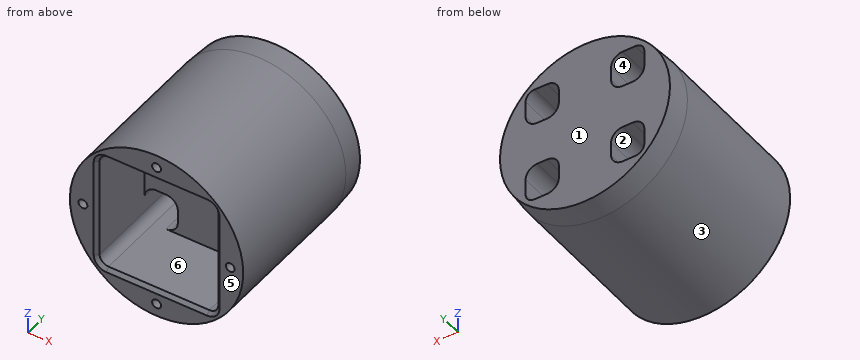
from build123d import *

# Parameters (mm, degrees)
SKETCH2_R           = 73.75
MAINDOUGHNUT_DEPTH  = 150
SKETCH3_R           = 3.81
CUT_EXTRUDE1_DEPTH  = 183.696811685
NOSECONETAPER_SIZE  = 20
NOSECONETAPER_SIZE2 = 1.398536239
PAYLOADSTOPS_DEPTH  = 90
FILLET1_R           = 10
FILLET2_R           = 10
FILLET3_R           = 10
CHAMFER1_SIZE       = 3


with BuildPart() as part:
    # Sketch2 → MainDoughnut (new body)
    with BuildSketch(Plane(origin=(0, 0, 0), x_dir=(1, 0, 0), z_dir=(0, 1, 0))):
        with Locations(Location((0, 0, 0), (0, 0, 270))):
            Circle(SKETCH2_R)
        with BuildLine():
            Line((42.87, -50.5), (-42.87, -50.5))
            ThreePointArc((-42.87, -50.5), (-48.26522474, -48.26522474), (-50.5, -42.87))
            Line((-50.5, -42.87), (-50.5, 42.87))
            ThreePointArc((-50.5, 42.87), (-48.26522474, 48.26522474), (-42.87, 50.5))
            Line((-42.87, 50.5), (42.87, 50.5))
            ThreePointArc((42.87, 50.5), (48.26522474, 48.26522474), (50.5, 42.87))
            Line((50.5, 42.87), (50.5, -42.87))
            ThreePointArc((50.5, -42.87), (48.26522474, -48.26522474), (42.87, -50.5))
        make_face(mode=Mode.SUBTRACT)
    extrude(amount=MAINDOUGHNUT_DEPTH)

    # Sketch3 → Cut-Extrude1 (cut, through all)
    with BuildSketch(Plane(origin=(0, 150, 0), x_dir=(1, 0, 0), z_dir=(0, 1, 0))):
        with Locations(Location((-62.711477498, 0, 0), (0, 0, 270))):
            Circle(SKETCH3_R)
        with Locations(Location((0, 62.711477498, 0), (0, 0, 270))):
            Circle(SKETCH3_R)
        with Locations(Location((62.711477498, 0, 0), (0, 0, 270))):
            Circle(SKETCH3_R)
        with Locations(Location((0, -62.711477498, 0), (0, 0, 270))):
            Circle(SKETCH3_R)
    extrude(amount=-CUT_EXTRUDE1_DEPTH, mode=Mode.SUBTRACT)

    # NoseconeTaper
    noseconetaper_edges = [part.edges().sort_by_distance(p)[0] for p in [
        (0, 150, -73.75),
    ]]
    noseconetaper_side = [part.faces().sort_by_distance(p)[0] for p in [
        (0, 75, -73.75),
    ]]
    chamfer(noseconetaper_edges, length=NOSECONETAPER_SIZE, length2=NOSECONETAPER_SIZE2, reference=noseconetaper_side[0])

    # Sketch5 → PayloadStops (add)
    with BuildSketch(Plane(origin=(0, 150, 0), x_dir=(1, 0, 0), z_dir=(0, 1, 0))):
        with BuildLine():
            Line((-22.25166399, 28.829478379), (-22.25166399, 68.844736604))
            Line((-22.25166399, 68.844736604), (22.25166399, 68.844736604))
            Line((22.25166399, 68.844736604), (22.25166399, 28.829478379))
            ThreePointArc((22.25166399, 28.829478379), (25.180596178, 21.758410568), (32.25166399, 18.829478379))
            Line((32.25166399, 18.829478379), (68.578942308, 18.829478379))
            Line((68.578942308, 18.829478379), (68.578942308, -18.829478379))
            Line((68.578942308, -18.829478379), (32.25166399, -18.829478379))
            ThreePointArc((32.25166399, -18.829478379), (25.180596178, -21.758410568), (22.25166399, -28.829478379))
            Line((22.25166399, -28.829478379), (22.25166399, -67.546162244))
            Line((22.25166399, -67.546162244), (-22.25166399, -67.546162244))
            Line((-22.25166399, -67.546162244), (-22.25166399, -28.829478379))
            ThreePointArc((-22.25166399, -28.829478379), (-25.180596178, -21.758410568), (-32.25166399, -18.829478379))
            Line((-32.25166399, -18.829478379), (-69.858321282, -18.829478379))
            Line((-69.858321282, -18.829478379), (-69.858321282, 18.829478379))
            Line((-69.858321282, 18.829478379), (-32.25166399, 18.829478379))
            ThreePointArc((-32.25166399, 18.829478379), (-25.180596178, 21.758410568), (-22.25166399, 28.829478379))
        make_face()
    extrude(amount=-PAYLOADSTOPS_DEPTH)

    # Fillet1
    fillet1_edges = [part.edges().sort_by_distance(p)[0] for p in [
        (-22.25166399, 105, -50.5),
    ]]
    fillet(fillet1_edges, radius=FILLET1_R)

    # Fillet2
    fillet2_edges = [part.edges().sort_by_distance(p)[0] for p in [
        (-50.5, 105, -18.829478379),
    ]]
    fillet(fillet2_edges, radius=FILLET2_R)

    # Fillet3
    fillet3_edges = [part.edges().sort_by_distance(p)[0] for p in [
        (50.5, 105, 18.829478379),
        (50.5, 105, -18.829478379),
        (-22.25166399, 105, 50.5),
        (22.25166399, 105, 50.5),
        (22.25166399, 105, -50.5),
        (-50.5, 105, 18.829478379),
    ]]
    fillet(fillet3_edges, radius=FILLET3_R)

    # Chamfer1
    chamfer1_edges = [part.edges().sort_by_distance(p)[0] for p in [
        (-48.26522474, 0, -48.26522474),
        (-50.5, 0, 0),
        (-48.26522474, 0, 48.26522474),
        (0, 0, 50.5),
        (48.26522474, 0, 48.26522474),
        (50.5, 0, 0),
        (48.26522474, 0, -48.26522474),
        (0, 0, -50.5),
    ]]
    chamfer(chamfer1_edges, length=CHAMFER1_SIZE)


solid = part.part
Read the model definition and answer for the solid it produces. Units are mm, in the model's axes. Face numbers are marked on the shaded views. A direction names the side the tool comes from. Round coordinates to 2 decimals unless told otherwise and drop trailing zeros. Write each loop counter-clockwise with the first axis right and the second up, starting at its lowest first coordinate (ties: lowest second). Pieces come first, ordered by that corner, then holes.
1. Which of the six approach directions +Z, -Z, +X, -X, +Y, -Y give full straight-line access (tool end or side, diameter ignored) to the marked faces 4, 5 and 6?
2. The part is cut by section D-D, the plane y = 24. Determine the outline of the cut face in (x, z), then the cut area to 3 significant figures.
3. The part is cut by section B-B, the plane x = 0. Determine the outline of the cut face in (y, z), then the cut area to 3 significant figures.
4. Straight lines are drawn through the part: L1, parallel to Z at x = 40.5, y = 69; L2, parallel to X at y = 17.5, z = 2.5; L3, parallel to X at y = 98.5, z = -47. For each, find the intervals that lie inside material, in ascending order.
5. Given pin 1 Ø2 at (x, y) = (-11.5, 59) entering from +Z; pin 2 Ø12 at (x, z) = (-3, -18) entering from -Y; pin 3 Ø6 at (x, y) = (-57, 82) entering from -Z, each flat-ended and moving along its own axis, determine where each tip first touches the part or whether it passes through.
6. The part is cut by section C-C, the plane z = 0. Determine the outline of the cut face in (x, y), then the cut area to 3 significant figures.
7. Determine the mould class of the marked faces 1, 2 and 3 for opening direction Z: pulls with the +Z half, pulls with the -Z half, needs draft (parallel to the pull), parting line crosses it, or undercut.
8. The part is cut by section A-A, the plane y = 127.5. State how many separate pieces and enclosed holes the cut face has, then the cut area to 3 significant figures.
Values:
1. face 4: +Y, -Y
1. face 5: +Z, -Z, +X, -X, -Y
1. face 6: -Y
2. outline: circle Ø147.5 at (0, 0); hole circle Ø7.62 at (-62.71, 0); hole (-50.5, -42.87) arc R7.63 ccw to (-42.87, -50.5) - (42.87, -50.5) arc R7.63 ccw to (50.5, -42.87) - (50.5, 42.87) arc R7.63 ccw to (42.87, 50.5) - (-42.87, 50.5) arc R7.63 ccw to (-50.5, 42.87) - close; hole circle Ø7.62 at (0, -62.71); hole circle Ø7.62 at (0, 62.71); hole circle Ø7.62 at (62.71, 0)
2. area: 6,750 mm2
3. outline: (0, -73.75) - (130, -73.75) - (150, -72.35) - (150, 72.35) - (130, 73.75) - (0, 73.75) - (0, 66.52) - (60, 66.52) - (60, 58.9) - (0, 58.9) - (0, 53.5) - (3, 50.5) - (60, 50.5) - (60, -50.5) - (3, -50.5) - (0, -53.5) - (0, -58.9) - (60, -58.9) - (60, -66.52) - (0, -66.52) - close
3. area: 15,100 mm2
4. L1: z = -61.63 to -50.5, -18.83 to 18.83, 50.5 to 61.63
4. L2: x = -73.71 to -65.59, -59.84 to -50.5, 50.5 to 59.84, 65.59 to 73.71
4. L3: x = -56.83 to -49.29, -24.65 to 24.65, 49.29 to 56.83
5. pin 1: stops at z = 73
5. pin 2: stops at y = 60
5. pin 3: stops at z = -50.23
6. outline: (-73.75, 0) - (-66.52, 0) - (-66.52, 60) - (-58.9, 60) - (-58.9, 0) - (-53.5, 0) - (-50.5, 3) - (-50.5, 60) - (50.5, 60) - (50.5, 3) - (53.5, 0) - (58.9, 0) - (58.9, 60) - (66.52, 60) - (66.52, 0) - (73.75, 0) - (73.75, 130) - (72.35, 150) - (-72.35, 150) - (-73.75, 130) - close
6. area: 15,100 mm2
7. face 1: needs draft
7. face 2: undercut
7. face 3: parting line crosses it
8. separate pieces: 1
8. enclosed holes: 4
8. area: 13,800 mm2
